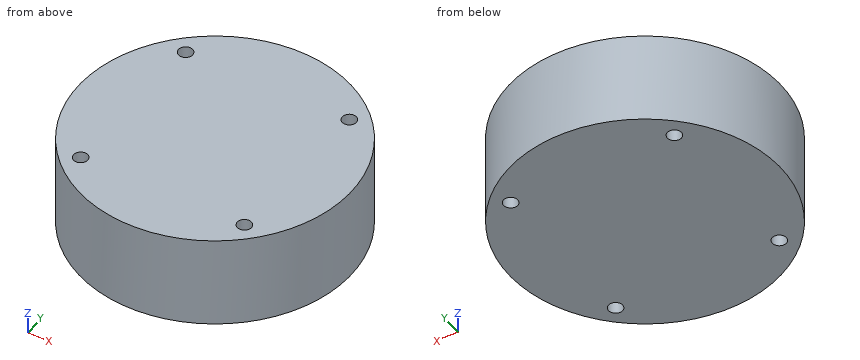
Autodesk Inventor part; units mm, degrees
ref_plane "YZ Plane" through (0, 0, 0) normal (1, 0, 0) x (0, 1, 0)
ref_plane "XZ Plane" through (0, 0, 0) normal (0, 1, 0) x (-1, 0, 0)
ref_plane "XY Plane" through (0, 0, 0) normal (0, 0, 1) x (1, 0, 0)
sketch "Sketch1" plane through (0, 0, 0) normal (0, 0, 1) x (1, 0, 0)
  line L0 (0, 55.4736) -> (0, -55.4736)
  line L1 (-55.4736, 0) -> (55.4736, 0)
  circle A0 centre (0, 0) radius 39.624
  circle A1 centre (0, 0) radius 10.3188
  dimension "d0" = 20.6375
  dimension "d1" = 79.248
extrude "Extrusion1" add sketch "Sketch1" along normal blind 26.924
sketch "Sketch2" plane through (0, 0, 0) normal (0, 0, -1) x (-1, 0, 0)
  line L0 (0, -55.4736) -> (0, 55.4736)
  line L1 (-55.4736, 0) -> (55.4736, 0)
  line L2 (-24.1554, -24.1554) -> (24.1554, -24.1554) construction
  line L3 (24.1554, -24.1554) -> (24.1554, 24.1554) construction
  line L4 (24.1554, 24.1554) -> (-24.1554, 24.1554) construction
  line L5 (-24.1554, 24.1554) -> (-24.1554, -24.1554) construction
  line L6 (-24.1554, -24.1554) -> (24.1554, 24.1554) construction
  line L7 (24.1554, -24.1554) -> (-24.1554, 24.1554) construction
  point P0 (0, 0)
  dimension "d22" = 48.3108
hole "Hole1" at (-24.1554, -24.1554, 0) direction (0, 0, 1) diameter 4.1402 depth 14.1986 tip angle 118
sketch "Sketch3" plane through (0, 0, 26.924) normal (0, 0, 1) x (1, 0, 0)
  circle A0 centre (-24.1554, -24.1554) radius 2.0701
  point P0 (0, 0)
hole "Hole2" at (-24.1554, -24.1554, 26.924) direction (0, 0, -1) diameter 4.1402 depth 14.1986 tip angle 118
pattern_circular "Circular Pattern1" count 4 over 360 about axis through (0, 0, -10) along (0, 0, 1) of "Hole1", "Hole2"
properties part number "J008109" material "ALUMINUM, 6061-T651"
Can you work these out from the model? Positions are in its coordinate system, mm. Coordinates: 2 decimals unless noted, no trailing zeros. Order: outer loops, then holes, each group sorted by start corner. A loop starts at its lowest first (then second) coordinate and runs counter-clockwise, first axis right, second up. Notation, with made-up numbers: (-28.5, 79.25) - (-0.5, 79.25) arc R7 ccw to (-0.5, 84.25) - close; hole circle Ø5 at (-33.75, 39). An arc over 180 degrees is marked (long way). Answer as a JSON object with one key per item and string values. Group by question number.
Q1. Imagine slicing it at C-C (y = -13). Please give me the cut outline in (x, z).
Q2. I need wall thicknesses on line 1 (X direction, y = -24, z = 7.5); line 2 (X direction, y = -24.5, z = 2.25); line 3 (Y direction, x = 1, z = 20.75). Which ranges of each line are inside material? Lowest first, please. Write a range as from..to.
Q3. Imagine slicing it at A-A (z = 6). Please give me the cut outline in (x, y), and give its area (3 significant figures).
Q4. Imagine slicing it at B-B (x = -27.5). Please give me the cut outline in (y, z), and give its area (3 significant figures).
Q5. Will these pins go through, and if not, where does the flat tip stop? P1, Ø3, axis at y = -9, z = 13, coming from the +X side; P2, Ø5, axis at x = 14, z = 13, coming from the +Y side; P3, Ø5, axis at y = 15.5, z = 14, coming from the +X side; P4, Ø3.5, axis at x = -24.16, y = 24.16, coming from the +Z side.
Determined:
{
 "1": {"outline": "(-37.43, 0) - (37.43, 0) - (37.43, 26.92) - (-37.43, 26.92) - close"},
 "2": {"line 1": "x = -31.53..-26.22, -22.09..22.09, 26.22..31.53", "line 2": "x = -31.14..-26.2, -22.11..22.11, 26.2..31.14", "line 3": "y = -39.61..39.61"},
 "3": {"outline": "circle Ø79.25 at (0, 0); hole circle Ø4.14 at (-24.16, -24.16); hole circle Ø4.14 at (-24.16, 24.16); hole circle Ø4.14 at (24.16, -24.16); hole circle Ø4.14 at (24.16, 24.16)", "area": "4,880 mm2"},
 "4": {"outline": "(-28.53, 0) - (28.53, 0) - (28.53, 26.92) - (-28.53, 26.92) - close", "area": "1,540 mm2"},
 "5": {"P1": "stops at x = 38.91", "P2": "stops at y = 37.92", "P3": "stops at x = 37.43", "P4": "passes through"}
}
